from build123d import *

# Parameters (mm, degrees)
F0_W         = 137.16
F0_H         = 37.338
F1_DEPTH     = 20.32
F2_W         = 130.048
F2_H         = 30.226
F3_DEPTH     = 11.43
F4_W         = 8.89
F4_H         = 21.844
F5_DEPTH     = 5.08
F6_T1_DEPTH  = 30.8870452561
F6_T3_DEPTH  = 52.8840905123
F6_T5_DEPTH  = 52.8840905123
F6_T7_DEPTH  = 52.8840905123
F6_T9_DEPTH  = 52.8840905123
F6_T11_DEPTH = 52.8840905123
F6_T13_DEPTH = 30.8870452561
F7_W         = 7.2538567698
F7_H         = 5.6681656279
F7_W_2       = 6.35
F8_DEPTH     = 5.08
F9_R         = 5.07999


# Not quite as in the source:
# - a fillet or chamfer that OpenCascade refuses, or shapes differently, is made with other operations: its cross-section is extruded or revolved along the edge and cut away or added
# - a fillet or chamfer is up to 0.001 mm smaller than in the source, because OpenCascade refuses the exact size
# - a feature names something its author has since deleted; it is built from what else it names


with BuildPart() as f1:
    # F0 (on Top) → F1 (new body)
    with BuildSketch(Plane.XY):
        Rectangle(F0_W, F0_H)
    extrude(amount=F1_DEPTH)

    # F2 (on face) → F3 (cut)
    with BuildSketch(Plane.XY.offset(20.32)):
        Rectangle(F2_W, F2_H)
    extrude(amount=-F3_DEPTH, mode=Mode.SUBTRACT)

    # F4 (on face) → F5 (join)
    with BuildSketch(Plane.XY.offset(8.89)):
        Rectangle(F4_W, F4_H)
        with Locations((15.24, 0)):
            Rectangle(F4_W, F4_H)
        with Locations((30.48, 0)):
            Rectangle(F4_W, F4_H)
        with Locations((45.72, 0)):
            Rectangle(F4_W, F4_H)
        with Locations((-15.24, 0)):
            Rectangle(F4_W, F4_H)
        with Locations((-30.48, 0)):
            Rectangle(F4_W, F4_H)
        with Locations((-45.72, 0)):
            Rectangle(F4_W, F4_H)
    extrude(amount=F5_DEPTH)

    # F6: fillet of radius 10.16 on 14 edges, made by hand

    # F6_s2 → F6_t1 (cut)
    with BuildSketch(Plane.YZ.offset(-50.165)):
        with BuildLine():
            ThreePointArc((-10.922, 8.89), (-7.2031818975, 12.6088181024), (-2.1231818975, 13.97))
            Line((-2.1231818975, 13.97), (-10.922, 13.97))
            Line((-10.922, 13.97), (-10.922, 8.89))
        make_face()
        with BuildLine():
            ThreePointArc((10.922, 8.89), (7.2031818975, 12.6088181024), (2.1231818975, 13.97))
            Line((2.1231818975, 13.97), (10.922, 13.97))
            Line((10.922, 13.97), (10.922, 8.89))
        make_face()
    extrude(amount=F6_T1_DEPTH, mode=Mode.SUBTRACT)

    # F6_s4 → F6_t3 (cut)
    with BuildSketch(Plane.YZ.offset(-56.9220452561)):
        with BuildLine():
            ThreePointArc((-10.922, 8.89), (-7.2031818975, 12.6088181024), (-2.1231818975, 13.97))
            Line((-2.1231818975, 13.97), (-10.922, 13.97))
            Line((-10.922, 13.97), (-10.922, 8.89))
        make_face()
        with BuildLine():
            ThreePointArc((10.922, 8.89), (7.2031818975, 12.6088181024), (2.1231818975, 13.97))
            Line((2.1231818975, 13.97), (10.922, 13.97))
            Line((10.922, 13.97), (10.922, 8.89))
        make_face()
    extrude(amount=F6_T3_DEPTH, mode=Mode.SUBTRACT)

    # F6_s6 → F6_t5 (cut)
    with BuildSketch(Plane.YZ.offset(-41.6820452561)):
        with BuildLine():
            ThreePointArc((-10.922, 8.89), (-7.2031818975, 12.6088181024), (-2.1231818975, 13.97))
            Line((-2.1231818975, 13.97), (-10.922, 13.97))
            Line((-10.922, 13.97), (-10.922, 8.89))
        make_face()
        with BuildLine():
            ThreePointArc((10.922, 8.89), (7.2031818975, 12.6088181024), (2.1231818975, 13.97))
            Line((2.1231818975, 13.97), (10.922, 13.97))
            Line((10.922, 13.97), (10.922, 8.89))
        make_face()
    extrude(amount=F6_T5_DEPTH, mode=Mode.SUBTRACT)

    # F6_s8 → F6_t7 (cut)
    with BuildSketch(Plane.YZ.offset(-26.4420452561)):
        with BuildLine():
            ThreePointArc((-10.922, 8.89), (-7.2031818975, 12.6088181024), (-2.1231818975, 13.97))
            Line((-2.1231818975, 13.97), (-10.922, 13.97))
            Line((-10.922, 13.97), (-10.922, 8.89))
        make_face()
        with BuildLine():
            ThreePointArc((10.922, 8.89), (7.2031818975, 12.6088181024), (2.1231818975, 13.97))
            Line((2.1231818975, 13.97), (10.922, 13.97))
            Line((10.922, 13.97), (10.922, 8.89))
        make_face()
    extrude(amount=F6_T7_DEPTH, mode=Mode.SUBTRACT)

    # F6_s10 → F6_t9 (cut)
    with BuildSketch(Plane.YZ.offset(-11.2020452561)):
        with BuildLine():
            ThreePointArc((-10.922, 8.89), (-7.2031818975, 12.6088181024), (-2.1231818975, 13.97))
            Line((-2.1231818975, 13.97), (-10.922, 13.97))
            Line((-10.922, 13.97), (-10.922, 8.89))
        make_face()
        with BuildLine():
            ThreePointArc((10.922, 8.89), (7.2031818975, 12.6088181024), (2.1231818975, 13.97))
            Line((2.1231818975, 13.97), (10.922, 13.97))
            Line((10.922, 13.97), (10.922, 8.89))
        make_face()
    extrude(amount=F6_T9_DEPTH, mode=Mode.SUBTRACT)

    # F6_s12 → F6_t11 (cut)
    with BuildSketch(Plane.YZ.offset(4.0379547439)):
        with BuildLine():
            ThreePointArc((-10.922, 8.89), (-7.2031818975, 12.6088181024), (-2.1231818975, 13.97))
            Line((-2.1231818975, 13.97), (-10.922, 13.97))
            Line((-10.922, 13.97), (-10.922, 8.89))
        make_face()
        with BuildLine():
            ThreePointArc((10.922, 8.89), (7.2031818975, 12.6088181024), (2.1231818975, 13.97))
            Line((2.1231818975, 13.97), (10.922, 13.97))
            Line((10.922, 13.97), (10.922, 8.89))
        make_face()
    extrude(amount=F6_T11_DEPTH, mode=Mode.SUBTRACT)

    # F6_s14 → F6_t13 (cut)
    with BuildSketch(Plane.YZ.offset(19.2779547439)):
        with BuildLine():
            ThreePointArc((-10.922, 8.89), (-7.2031818975, 12.6088181024), (-2.1231818975, 13.97))
            Line((-2.1231818975, 13.97), (-10.922, 13.97))
            Line((-10.922, 13.97), (-10.922, 8.89))
        make_face()
        with BuildLine():
            ThreePointArc((10.922, 8.89), (7.2031818975, 12.6088181024), (2.1231818975, 13.97))
            Line((2.1231818975, 13.97), (10.922, 13.97))
            Line((10.922, 13.97), (10.922, 8.89))
        make_face()
    extrude(amount=F6_T13_DEPTH, mode=Mode.SUBTRACT)

    # F7 (on face) → F8 (join)
    with BuildSketch(Plane.XY.offset(8.89)):
        with Locations((-53.7919283849, 0)):
            Rectangle(F7_W, F7_H)
        with Locations((-38.1, 0)):
            Rectangle(F7_W_2, F7_H)
        with Locations((-22.86, 0)):
            Rectangle(F7_W_2, F7_H)
        with Locations((-7.62, 0)):
            Rectangle(F7_W_2, F7_H)
        with Locations((7.62, 0)):
            Rectangle(F7_W_2, F7_H)
        with Locations((22.86, 0)):
            Rectangle(F7_W_2, F7_H)
        with Locations((38.1, 0)):
            Rectangle(F7_W_2, F7_H)
        with Locations((53.7919283849, 0)):
            Rectangle(F7_W, F7_H)
    extrude(amount=F8_DEPTH)

    # F9 (radius 5.08 in the source; OpenCascade refuses exactly that, so slightly less here)
    f9_edges = [f1.edges().sort_by_distance(p)[0] for p in [
        (-57.418857, 0, 13.97),
        (57.418857, 0, 13.97),
    ]]
    fillet(f9_edges, radius=F9_R)


solid = f1.part
The listing builds one solid part. Answer for the finished solid, in the listing's coordinates (mm). A direction names the side the tool comes from. Round coordinates to 2 decimals unless told otherwise and drop trailing zeros. Order: outer loops, then holes, each group sorted by start corner. A loop starts at its lowest first (then second) coordinate and runs counter-clockwise, first axis right, second up. Notation, with made-up numbers: (20, -6) - (31, -6) arc R7 ccw to (31, 2) - close; hole circle Ø8 at (41, -15). An arc over 180 degrees is marked (long way). Write item = value, one per line. Start each with the question number.
1) For a pull along X with two mould halves and no side action, classify faces 3 (the flat face through (-1, 0, 0)), 4 (the cylindrical face through (55.89, 0.04, 12.52)), 5 (the flat face through (8, 2.834, 11)), 6 (the flat face through (-68.58, 0, 10)) as released by +X, released by -X, zero draft, split by the parting line, or undercut.
2) Section C-C, the plane x = -45 is taken. Write down the section's boundary in (y, z).
3) Section D-D, the plane z = 11 is taken. Count the separate pieces of the cut face and the enclosed holes in it, plus the area to 3 significant figures.
4) Straight lines are drawn through the part: L1, parallel to Y at x = -23.5, z = 12; L2, parallel to X at y = -4, z = 16.5; L3, parallel to Y at x = -52, z = 15.25. For each, find the intervals that lie inside material, in ascending order.
5) For faces 1 (the flat face through (-1, 18.669, 10)), 2 (the cylindrical face through (-55.97, 0.04, 12.44)), determine the directions among +Z, -Z, +X, -X, +Y, -Y from which every point of the face is accessible in a straight line to the end or side of a thin tool.
6) Section B-B, the plane y = -13 is taken. Write down the section's boundary in (x, z), plus the area to 3 significant figures.
7) Given pin 1 (5 mm diameter, centred on x = -11, y = 7.5, fed in from +Z); pin 2 (1 mm diameter, centred on x = 40, y = 3, fed in from +Z), each flat-ended and moving along its own axis, determine where each tip first touches the part or whether it passes through.
8) Section A-A, the plane z = 17.75 is taken. Write down the section's boundary in (x, y).
Results list:
q1.face_3 = zero draft
q1.face_4 = undercut
q1.face_5 = undercut
q1.face_6 = released by -X
q2.outline = (-18.67, 0) - (18.67, 0) - (18.67, 20.32) - (15.11, 20.32) - (15.11, 8.89) - (10.92, 8.89) arc R10.16 ccw to (2.12, 13.97) - (-2.12, 13.97) arc R10.16 ccw to (-10.92, 8.89) - (-15.11, 8.89) - (-15.11, 20.32) - (-18.67, 20.32) - close
q3.separate_pieces = 2
q3.enclosed_holes = 1
q3.area = 2,640 mm^2
q4.L1 = -18.67 to -15.11, -2.83 to 2.83, 15.11 to 18.67
q4.L2 = -68.58 to -65.02, 65.02 to 68.58
q4.L3 = -18.67 to -15.11, 15.11 to 18.67
q5.face_1 = +Z, -Z, +X, -X, +Y
q5.face_2 = +Z
q6.outline = (-68.58, 0) - (68.58, 0) - (68.58, 20.32) - (65.02, 20.32) - (65.02, 8.89) - (-65.02, 8.89) - (-65.02, 20.32) - (-68.58, 20.32) - close
q6.area = 1,300 mm^2
q7.pin_1 = 13.55
q7.pin_2 = 13.97
q8.outline = (-68.58, -18.67) - (68.58, -18.67) - (68.58, 18.67) - (-68.58, 18.67) - close; hole (-65.02, -15.11) - (65.02, -15.11) - (65.02, 15.11) - (-65.02, 15.11) - close
